Source: CAD feature listing. Evaluate the final solid. Frame: model axes, mm. Face numbers are marked on the shaded views. Coordinates: 2 decimals unless noted, no trailing zeros. Loops run counter-clockwise (first coordinate to the right, second up) from the corner with the lowest first, then second, coordinate; pieces in that order, holes last.
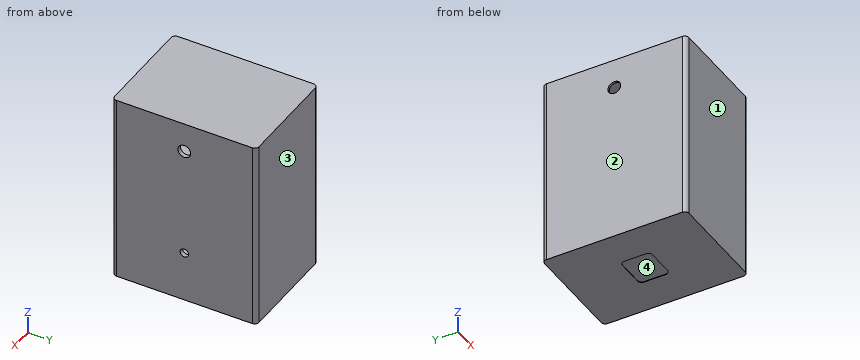
from build123d import *

# Parameters (mm, degrees)
SKETCH_1_W          = 250
SKETCH_1_H          = 340.4
EXTRUDE_1_DEPTH     = 450
FILLET_1_R          = 10
SKETCH_4_R          = 10
CUT_EXTRUDE_1_DEPTH = 50
CUT_EXTRUDE_2_DEPTH = 1
CUT_EXTRUDE_START   = -5
CUT_EXTRUDE_3_DEPTH = 440
SKETCH_8_R          = 15
CUT_EXTRUDE_4_DEPTH = 543.188196109
EXTRUDE_START       = -5
SKETCH_11_W         = 8
SKETCH_11_H         = 320.4
EXTRUDE_2_DEPTH     = 235


with BuildPart() as part:
    # 草图1 → 凸台-拉伸1 (new body)
    with BuildSketch(Plane.XY):
        Rectangle(SKETCH_1_W, SKETCH_1_H)
    extrude(amount=EXTRUDE_1_DEPTH)

    # 圆角1
    fillet_1_edges = [part.edges().sort_by_distance(p)[0] for p in [
        (125, -170.2, 225),
        (-125, -170.2, 225),
        (-125, 170.2, 225),
        (125, 170.2, 225),
    ]]
    fillet(fillet_1_edges, radius=FILLET_1_R)

    # 草图4 → 切除-拉伸1 (cut)
    with BuildSketch(Plane(origin=(125, 0, 0), x_dir=(0, 0, -1), z_dir=(1, 0, 0))):
        with Locations(Location((-120, 0, 0), (0, 0, 270))):
            Circle(SKETCH_4_R)
    extrude(amount=-CUT_EXTRUDE_1_DEPTH, mode=Mode.SUBTRACT)

    # 草图5 → 切除-拉伸2 (cut)
    with BuildSketch(Plane(origin=(0, 0, 0), x_dir=(-1, 0, 0), z_dir=(0, 0, -1))):
        with BuildLine():
            Line((-30.5, -35.5), (30.5, -35.5))
            ThreePointArc((30.5, -35.5), (37.571067812, -32.571067812), (40.5, -25.5))
            Line((40.5, -25.5), (40.5, 25.5))
            ThreePointArc((40.5, 25.5), (37.571067812, 32.571067812), (30.5, 35.5))
            Line((30.5, 35.5), (-30.5, 35.5))
            ThreePointArc((-30.5, 35.5), (-37.571067812, 32.571067812), (-40.5, 25.5))
            Line((-40.5, 25.5), (-40.5, -25.5))
            ThreePointArc((-40.5, -25.5), (-37.571067812, -32.571067812), (-30.5, -35.5))
        make_face()
    extrude(amount=-CUT_EXTRUDE_2_DEPTH, mode=Mode.SUBTRACT)

    # 草图7 → 切除-拉伸3 (cut)
    with BuildSketch(Plane.XY.offset(450).offset(CUT_EXTRUDE_START)):
        Polygon((-120, -160.2), (-120, 160.2), (115, 160.2), (115, -160.2), (-18.295526733, -160.2), align=None)
    extrude(amount=-CUT_EXTRUDE_3_DEPTH, mode=Mode.SUBTRACT)

    # 草图8 → 切除-拉伸4 (cut, through all)
    with BuildSketch(Plane.ZY.offset(125)):
        with Locations(Location((380, 0, 0), (0, 0, 270))):
            Circle(SKETCH_8_R)
    extrude(amount=-CUT_EXTRUDE_4_DEPTH, mode=Mode.SUBTRACT)

    # 草图11 → 凸台-拉伸2 (add)
    with BuildSketch(Plane(origin=(125, 0, 0), x_dir=(0, 0, -1), z_dir=(1, 0, 0)).offset(EXTRUDE_START)):
        with Locations((-326, 0)):
            Rectangle(SKETCH_11_W, SKETCH_11_H)
    extrude(amount=-EXTRUDE_2_DEPTH)


solid = part.part
Q1. Line query: line 1 along Z through (x, y) = (68, 115); line 2 along Z through (x, y) = (122, 0); line 3 along X through (y, z) = (-33, 396.5). Output: solid intervals per line, ascending.
Q2. Section A-A, the plane y = 0. Return the cut outline in (x, z), plus the area to 3 significant figures.
Q3. Section B-B, the plane x = -21. Return the cut outline in (y, z).
Q4. Section C-C, the plane z = 356.5. Return the cut outline in (x, y), plus the area to 3 significant figures.
Q5. Draft query along Y for the marked faces 1, 2, 3 and 4. Return one class per face: +Y half, -Y half, draft (parallel to the pull), parting line (faces both ways), or undercut.
Q6. Section D-D, the plane y = -70. Return the cut outline in (x, z).
Q7. Contact query for a flat-ended pin moving along its axis: pin 1 Ø21.5 at (x, y) = (-10, 9.5) entering from -Z. Output: stop coordinate, or through.
Derived:
1. line 1: z = 0 to 5, 322 to 330, 445 to 450
1. line 2: z = 0 to 110, 130 to 365, 395 to 450
1. line 3: x = -125 to -120, 115 to 125
2. outline: (-125, 0) - (-40.5, 0) - (-40.5, 1) - (40.5, 1) - (40.5, 0) - (125, 0) - (125, 110) - (115, 110) - (115, 5) - (-120, 5) - (-120, 365) - (-125, 365) - close; (-125, 395) - (-120, 395) - (-120, 445) - (115, 445) - (115, 395) - (125, 395) - (125, 450) - (-125, 450) - close; (-115, 322) - (115, 322) - (115, 130) - (125, 130) - (125, 365) - (115, 365) - (115, 330) - (-115, 330) - close
2. area: 10,200 mm2
3. outline: (-170.2, 0) - (-35.5, 0) - (-35.5, 1) - (35.5, 1) - (35.5, 0) - (170.2, 0) - (170.2, 450) - (-170.2, 450) - close; hole (-160.2, 5) - (160.2, 5) - (160.2, 322) - (-160.2, 322) - close; hole (-160.2, 330) - (160.2, 330) - (160.2, 445) - (-160.2, 445) - close
4. outline: (-125, -160.2) arc R10 ccw to (-115, -170.2) - (115, -170.2) arc R10 ccw to (125, -160.2) - (125, 160.2) arc R10 ccw to (115, 170.2) - (-115, 170.2) arc R10 ccw to (-125, 160.2) - close; hole (-120, -160.2) - (115, -160.2) - (115, 160.2) - (-120, 160.2) - close
4. area: 9,720 mm2
5. face 1: -Y half
5. face 2: draft
5. face 3: +Y half
5. face 4: undercut
6. outline: (-125, 0) - (125, 0) - (125, 450) - (-125, 450) - close; hole (-120, 5) - (115, 5) - (115, 322) - (-115, 322) - (-115, 330) - (115, 330) - (115, 445) - (-120, 445) - close
7. pin 1: stops at z = 1
